```python
from build123d import *

# Parameters (mm, degrees)
F0_R     = 12.71
F1_DEPTH = 4.07
F2_R     = 5.5707205992
F3_DEPTH = 11.22
F4_R     = 2.9226210924
F5_DEPTH = 4.12
F6_R     = 2.375
F7_DEPTH = 3.02


with BuildPart() as f1:
    # F0 (on Front) → F1 (new body)
    with BuildSketch(Plane.XZ):
        Circle(F0_R)
    extrude(amount=F1_DEPTH)

    # F2 (on Front) → F3 (join)
    with BuildSketch(Plane.XZ):
        Circle(F2_R)
    extrude(amount=F3_DEPTH)

    # F4 (on face) → F5 (join)
    with BuildSketch(Plane.XZ.offset(11.22)):
        Circle(F4_R)
    extrude(amount=F5_DEPTH)

    # F6 (on face) → F7 (cut, symmetric)
    with BuildSketch(Plane.XZ):
        Circle(F6_R)
    extrude(amount=F7_DEPTH, both=True, mode=Mode.SUBTRACT)


solid = f1.part
```
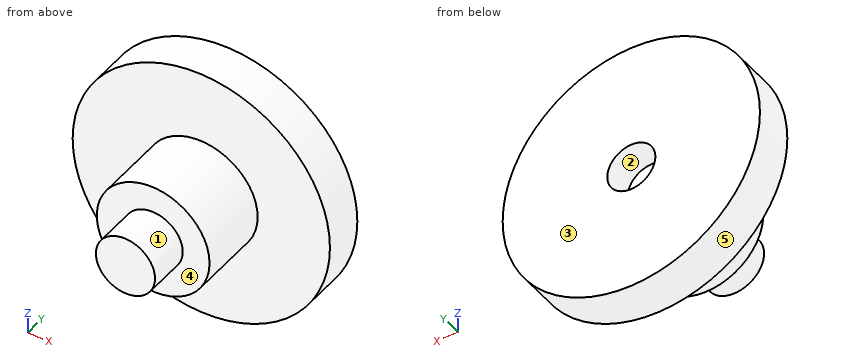
Verification items for the finished model (mm, model axes). Face numbers are marked on the shaded views. A direction names the side the tool comes from. Give positions to 0.01 mm unless a question says otherwise; leave off trailing zeros. Loops run counter-clockwise (first coordinate to the right, second up) from the corner with the lowest first, then second, coordinate; pieces in that order, holes last. Notation, with made-up numbers: M 26.25,38 L 70.25,38 A31 ccw 70.25,70 Z; hole C 49.25,-17 d9. An arc over 180 degrees is marked long. One line per question, with ' | ' between items.
Item 1: Draft check along X on the marked faces 1, 2 and 3. Enter one of: +X half, -X half, draft (parallel to the pull), parting line (faces both ways), or undercut.
Completed:
face 1: parting line | face 2: undercut | face 3: draft
Item 2: Section check D-D, the plane y = -5.5. Record the cut outline in (x, z), plus the area to 3 significant figures.
Completed:
outline: C 0,0 d11.14 | area: 97.5 mm^2
Item 3: Section check C-C, the plane y = -2.25. Record the cut outline in (x, z) (3 decimals), plus the area to 3 significant figures.
Completed:
outline: C 0,0 d25.42; hole C 0,0 d4.75 | area: 490 mm^2
Item 4: Section check B-B, the plane z = 0. Record the cut outline in (x, y) (3 decimals), plus the area to 3 significant figures.
Completed:
outline: M -12.71,-4.07 L -5.571,-4.07 L -5.571,-11.22 L -2.923,-11.22 L -2.923,-15.34 L 2.923,-15.34 L 2.923,-11.22 L 5.571,-11.22 L 5.571,-4.07 L 12.71,-4.07 L 12.71,0 L 2.375,0 L 2.375,-3.02 L -2.375,-3.02 L -2.375,0 L -12.71,0 Z | area: 193 mm^2
Item 5: Depth check by flat-ended pin: P1, Ø2, axis at x = 1, z = -3, coming from the -Y side; P2, Ø1, axis at y = -10, z = 0, coming from the +X side; P3, Ø4, axis at x = 0, z = 0, coming from the +Y side; P4, Ø1.5, axis at y = -7, z = -4, coming from the +X side. Enter the tip coordinate at first touch or a pass-through.
Completed:
P1: stops at y = -15.34 | P2: stops at x = 5.57 | P3: stops at y = -3.02 | P4: stops at x = 4.52
Item 6: Thickness scan on line 1 (Z direction, x = 0, y = -2.3) (3 decimals); line 2 (Y direction, x = -7.5, z = -3.75); line 3 (Y direction, x = -1.25, z = 0.5). Record the ranges inside material, lowest first. Write a range as [from, to].
Completed:
line 1: z = [-12.71, -2.375], [2.375, 12.71] | line 2: y = [-4.07, 0] | line 3: y = [-15.34, -3.02]
Item 7: Tool access check on the marked faces 4 and 5. Record the directions out of +Z, -Z, +X, -X, +Y, -Y that give a thin tool (end or side, any length) a straight path to the whole face; none if there is none.
Completed:
face 4: -Y | face 5: +Y, -Y
Item 8: Section check A-A, the plane x = 0. Record the cut outline in (y, z) (3 decimals), plus the area to 3 significant figures.
Completed:
outline: M -15.34,-2.923 L -11.22,-2.923 L -11.22,-5.571 L -4.07,-5.571 L -4.07,-12.71 L 0,-12.71 L 0,-2.375 L -3.02,-2.375 L -3.02,2.375 L 0,2.375 L 0,12.71 L -4.07,12.71 L -4.07,5.571 L -11.22,5.571 L -11.22,2.923 L -15.34,2.923 Z | area: 193 mm^2
